from build123d import *

# Parameters (mm, degrees)
F0_W     = 19.05
F0_H     = 50.8
F1_DEPTH = 14.2875
F2_T     = -3.175
F4_D     = 4.826
F5_SIZE2 = 7.62
F5_SIZE  = 12.7


with BuildPart() as f1:
    # F0 (on Front) → F1 (new body, symmetric)
    with BuildSketch(Plane.XZ):
        with Locations((1.503078, -4.818475)):
            Rectangle(F0_W, F0_H)
    extrude(amount=F1_DEPTH, both=True)

    # F2
    f2_openings = [f1.faces().sort_by_distance(p)[0] for p in [
        (-8.021922, 0, -4.818475),
        (1.503078, 0, -30.218475),
        (1.503078, 14.2875, -4.818475),
        (1.503078, 0, 20.581525),
    ]]
    offset(amount=F2_T, openings=f2_openings)

    # F4 (through all)
    with Locations(Plane.YZ.offset(11.028078)):
        with Locations((3.4925, -4.818475)):
            Hole(F4_D / 2)

    # F5
    f5_edges = [f1.edges().sort_by_distance(p)[0] for p in [
        (9.440578, 14.2875, -30.218475),
        (9.440578, 14.2875, 20.581525),
    ]]
    chamfer(f5_edges, length=F5_SIZE, length2=F5_SIZE2)


solid = f1.part
Design review of the part built by this model. Coordinates are the model's own, in mm. A direction names the side the tool comes from. Round coordinates to 2 decimals unless told otherwise and drop trailing zeros. Write each loop counter-clockwise with the first axis right and the second up, starting at its lowest first coordinate (ties: lowest second). Pieces come first, ordered by that corner, then holes.
Item 1: Consider section C-C on y = -10. Give the boundary of the cut face in (x, z).
Item 2: For faces 4 (the flat face through (7.853, -1, -5)), 5 (the flat face through (9, 14.288, -5)), list the 3-axis set-ups (+Z, -Z, +X, -X, +Y, -Y) from which the entire face can be reached by the end or side of a thin tool; tool diameter is ignored.
Item 3: Consider section A-A on z = -4. Give the boundary of the cut face in (x, y).
Item 4: For pin 1 Ø5 at (x, z) = (-0.5, -13.5) entering from +Y; pin 2 Ø4.5 at (y, z) = (3.49, -4.82) entering from -X; pin 3 Ø2 at (y, z) = (-2, -3.5) entering from -X, all flat-tipped, find the tip position at first contact; note any pin that passes through.
Item 5: Wall thickness on L1, parallel to X at y = 4.75, z = -1; L2, parallel to Y at x = 4.5, z = -4; L3, parallel to Y at x = 8, z = -7: over which ranges is each line inside the solid? List them lowest first.
Item 6: Draft analysis for pull direction Z (two halves, no side actions). For faces 1 (the flat face through (1, -14.288, -4)), 2 (the cylindrical face through (9.418, 5.271, -3.188)), 3 (the flat face through (4, -13, 20.582)), state which applies: released by +Z, released by -Z, zero draft, split by the parting line, or undercut.
Item 7: Consider section B-B on x = 9. Give the boundary of the cut face in (y, z), and give its area (3 significant figures).
Item 8: Consider section D-D on x = 2. Give the boundary of the cut face in (y, z).
Check values:
1. outline: (7.85, -30.22) - (11.03, -30.22) - (11.03, 20.58) - (7.85, 20.58) - close
2. face 4: +Z, -Z, -X, +Y
2. face 5: +Z, -Z, +X, -X, +Y
3. outline: (-8.02, -14.29) - (11.03, -14.29) - (11.03, 1.22) - (7.85, 1.22) - (7.85, -11.11) - (-8.02, -11.11) - close; (7.85, 5.76) - (11.03, 5.76) - (11.03, 14.29) - (7.85, 14.29) - close
4. pin 1: stops at y = -11.11
4. pin 2: passes through
4. pin 3: stops at x = 7.85
5. L1: x = 7.85 to 11.03
5. L2: y = -14.29 to -11.11
5. L3: y = -14.29 to 2.46, 4.52 to 14.29
6. face 1: zero draft
6. face 2: undercut
6. face 3: released by +Z
7. outline: (-14.29, -30.22) - (1.59, -30.22) - (14.29, -22.6) - (14.29, 12.96) - (1.59, 20.58) - (-14.29, 20.58) - close; hole circle Ø4.83 at (3.49, -4.82)
7. area: 1,340 mm2
8. outline: (-14.29, -30.22) - (-11.11, -30.22) - (-11.11, 20.58) - (-14.29, 20.58) - close
